from build123d import *

# Parameters (mm, degrees)
PAD_DEPTH = 50
FILLET_R  = 0.35


with BuildPart() as part:
    # Sketch → Pad (new body)
    with BuildSketch(Plane.XZ):
        Polygon((-5.4, 0), (5.4, 0), (6, 0.6), (6, 3.8), (4.55, 5.25), (4.55, 5.65), (6, 7.1), (6, 7.4), (5.4, 8), (-5.4, 8), (-6, 7.4), (-6, 7.1), (-4.55, 5.65), (-4.55, 5.25), (-6, 3.8), (-6, 0.6), align=None)
    extrude(amount=PAD_DEPTH)

    # Fillet
    fillet_edges = [part.edges().sort_by_distance(p)[0] for p in [
        (0, 0, 0),
        (5.7, 0, 0.3),
        (6, 0, 2.2),
        (5.275, 0, 4.525),
        (4.55, 0, 5.45),
        (5.275, 0, 6.375),
        (6, 0, 7.25),
        (5.7, 0, 7.7),
        (0, 0, 8),
        (-5.7, 0, 7.7),
        (-6, 0, 7.25),
        (-5.275, 0, 6.375),
        (-4.55, 0, 5.45),
        (-5.275, 0, 4.525),
        (-6, 0, 2.2),
        (-5.7, 0, 0.3),
        (0, -50, 0),
        (5.7, -50, 0.3),
        (6, -50, 2.2),
        (5.275, -50, 4.525),
        (4.55, -50, 5.45),
        (5.275, -50, 6.375),
        (6, -50, 7.25),
        (5.7, -50, 7.7),
        (0, -50, 8),
        (-5.7, -50, 7.7),
        (-6, -50, 7.25),
        (-5.275, -50, 6.375),
        (-4.55, -50, 5.45),
        (-5.275, -50, 4.525),
        (-6, -50, 2.2),
        (-5.7, -50, 0.3),
    ]]
    fillet(fillet_edges, radius=FILLET_R)


solid = part.part
Work out the finished part from the listing and answer in its coordinate system (mm). A direction names the side the tool comes from. Give positions to 0.01 mm unless a question says otherwise; leave off trailing zeros. Loops run counter-clockwise (first coordinate to the right, second up) from the corner with the lowest first, then second, coordinate; pieces in that order, holes last. Notation, with made-up numbers: (82, 1) -> (105, 1) arc R23 cw to (105, 34) -> close; hole circle Ø6 at (-30, -3). An arc over 180 degrees is marked (long way). Use a Markdown table: item, result. Add a question column.
1. A flat-ended cylindrical pin translates along its axis: pin 1 Ø1.5 at (y, z) = (-34, 5.5) entering from +X. Find the tip coordinate at first contact, or state that the pin passes through.
2. Find the intervals of material crossed by probe 1 along Z at (x, y) = (5.25, -33.5); probe 2 along Z at (x, y) = (5.5, -13.5); probe 3 along X at (y, z) = (-44, 4), in increasing order.
3. For faces 1 (the flat face through (5.3, -24.7, 4.5)), 2 (the cylindrical face through (-5.142, -0.105, 6.383)), 3 (the flat face through (-5.3, -24.7, 4.5)), 4 (the cylindrical face through (5.142, -49.895, 4.517)), 5 (the cylindrical face through (-5.142, -49.895, 6.383)), determine the directions among +Z, -Z, +X, -X, +Y, -Y from which every point of the face is accessible in a straight line to the end or side of a thin tool.
4. Section A-A on y = -7 is taken. Determine the outline of the cut face in (x, z).
Results below:
| question | item | result |
|---|---|---|
| 1 | pin 1 | stops at x = 5.15 |
| 2 | probe 1 | z = 0 to 4.55, 6.35 to 8 |
| 2 | probe 2 | z = 0.1 to 4.3, 6.6 to 7.9 |
| 2 | probe 3 | x = -5.8 to 5.8 |
| 3 | face 1 | +X, +Y, -Y |
| 3 | face 2 | -X, +Y |
| 3 | face 3 | -X, +Y, -Y |
| 3 | face 4 | +X, -Y |
| 3 | face 5 | -X, -Y |
| 4 | outline | (-6, 0.6) -> (-5.4, 0) -> (5.4, 0) -> (6, 0.6) -> (6, 3.8) -> (4.55, 5.25) -> (4.55, 5.65) -> (6, 7.1) -> (6, 7.4) -> (5.4, 8) -> (-5.4, 8) -> (-6, 7.4) -> (-6, 7.1) -> (-4.55, 5.65) -> (-4.55, 5.25) -> (-6, 3.8) -> close |
